Design review of the part built by this model. Coordinates are the model's own, in mm. Face numbers are marked on the shaded views. A direction names the side the tool comes from. Coordinates: 2 decimals unless noted, no trailing zeros. Write each loop counter-clockwise with the first axis right and the second up, starting at its lowest first coordinate (ties: lowest second). Pieces come first, ordered by that corner, then holes. Notation, with made-up numbers: (73.25, 4.5) - (102.25, 4.5) arc R10 ccw to (102.25, 15.5) - close; hole circle Ø1 at (65.25, 88.25). An arc over 180 degrees is marked (long way). Use a Markdown table: item, result.
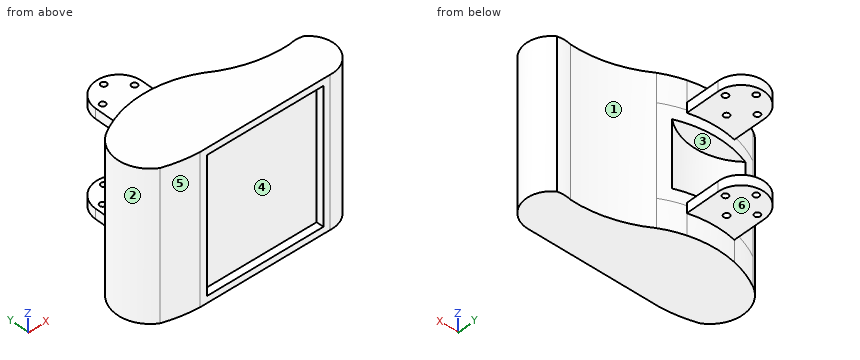
from build123d import *

# Parameters (mm, degrees)
BOSS_EXTRUDE1_DEPTH = 40
BOSS_EXTRUDE2_START = -1.2
BOSS_EXTRUDE2_DEPTH = 4.375
CUT_EXTRUDE2_START  = -29
CUT_EXTRUDE2_DEPTH  = 29
SKETCH10_R          = 1.25
CUT_EXTRUDE4_DEPTH  = 10
BOSS_EXTRUDE3_DEPTH = 12.5
SKETCH5_W           = 51.025429481
SKETCH5_H           = 59
CUT_EXTRUDE3_DEPTH  = 3.175


with BuildPart() as part:
    # Sketch1 → Boss-Extrude1 (new body)
    with BuildSketch(Plane.XY):
        with BuildLine():
            Line((-15, -2.886329782), (42.025429481, -2.886329782))
            ThreePointArc((42.025429481, -2.886329782), (53.05879951, 4.537892473), (48.73397068, 17.113670218))
            ThreePointArc((48.73397068, 17.113670218), (45.721020148, 17.497008544), (42.708069616, 17.113670218))
            ThreePointArc((42.708069616, 17.113670218), (27.113259503, 18.919115101), (12.833158081, 25.441111501))
            ThreePointArc((12.833158081, 25.441111501), (-8.642012727, 30.909979938), (-30, 25))
            ThreePointArc((-30, 25), (-37.166841919, 12.5), (-30, 0))
            ThreePointArc((-30, 0), (-22.60067635, -1.966370959), (-15, -2.886329782))
        make_face()
    extrude(amount=BOSS_EXTRUDE1_DEPTH)

    # Sketch3 → Boss-Extrude2 (add)
    with BuildSketch(Plane.XY.offset(40).offset(BOSS_EXTRUDE2_START)):
        with BuildLine():
            Line((-17.166841919, 44.092125176), (-17.166841919, 16.592125176))
            Line((-17.166841919, 16.592125176), (3.120389758, 16.592125176))
            Line((3.120389758, 16.592125176), (3.120389758, 44.092125176))
            ThreePointArc((3.120389758, 44.092125176), (-7.02322608, 54.235741015), (-17.166841919, 44.092125176))
        make_face()
    boss_extrude2 = extrude(amount=BOSS_EXTRUDE2_DEPTH)

    # Sketch4 → Cut-Extrude2 (cut)
    with BuildSketch(Plane.XY.offset(34.4).offset(CUT_EXTRUDE2_START)):
        with BuildLine():
            ThreePointArc((-23.782802313, 27.999798652), (-7.894532573, 21.994601327), (8.097551753, 27.717603087))
            ThreePointArc((8.097551753, 27.717603087), (-7.81561096, 30.910577643), (-23.782802313, 27.999798652))
        make_face()
    extrude(amount=CUT_EXTRUDE2_DEPTH, mode=Mode.SUBTRACT)

    # Sketch10 → Cut-Extrude4 (cut)
    with BuildSketch(Plane.XY.offset(43.175)):
        with Locations((-7.02322608, 51.235741015)):
            Circle(SKETCH10_R)
        with Locations((-0.02322608, 44.235741015)):
            Circle(SKETCH10_R)
        with Locations((-7.02322608, 37.235741015)):
            Circle(SKETCH10_R)
        with Locations((-14.02322608, 44.235741015)):
            Circle(SKETCH10_R)
    cut_extrude4 = extrude(amount=-CUT_EXTRUDE4_DEPTH, mode=Mode.SUBTRACT)

    # Sketch6 → Boss-Extrude3 (add)
    with BuildSketch(Plane.XY.offset(40)):
        with BuildLine():
            ThreePointArc((12.833158081, 25.441111501), (8.097551753, 27.717603087), (3.120389758, 29.401717013))
            Line((3.120389758, 29.401717013), (3.120389758, 16.592125176))
            Line((3.120389758, 16.592125176), (-17.166841919, 16.592125176))
            Line((-17.166841919, 16.592125176), (-17.166841919, 29.969927353))
            ThreePointArc((-17.166841919, 29.969927353), (-23.782802313, 27.999798652), (-30, 25))
            ThreePointArc((-30, 25), (-37.166841919, 12.5), (-30, 0))
            ThreePointArc((-30, 0), (-22.60067635, -1.966370959), (-15, -2.886329782))
            Line((-15, -2.886329782), (42.025429481, -2.886329782))
            ThreePointArc((42.025429481, -2.886329782), (53.05879951, 4.537892473), (48.73397068, 17.113670218))
            ThreePointArc((48.73397068, 17.113670218), (45.721020148, 17.497008544), (42.708069616, 17.113670218))
            ThreePointArc((42.708069616, 17.113670218), (27.113259503, 18.919115101), (12.833158081, 25.441111501))
        make_face()
        with BuildLine():
            Line((3.120389758, 16.592125176), (3.120389758, 29.401717013))
            ThreePointArc((3.120389758, 29.401717013), (-6.989349265, 30.895351044), (-17.166841919, 29.969927353))
            Line((-17.166841919, 29.969927353), (-17.166841919, 16.592125176))
            Line((-17.166841919, 16.592125176), (3.120389758, 16.592125176))
        make_face()
    boss_extrude3 = extrude(amount=BOSS_EXTRUDE3_DEPTH)

    # Mirror4: Boss-Extrude3 across plane
    add(boss_extrude3.mirror(Plane(origin=(0, 0, 20), x_dir=(1, 0, 0), z_dir=(0, 0, -1))))

    # Sketch5 → Cut-Extrude3 (cut)
    with BuildSketch(Plane.XZ.offset(2.886329782)):
        with Locations((13.512714741, 20)):
            Rectangle(SKETCH5_W, SKETCH5_H)
    extrude(amount=-CUT_EXTRUDE3_DEPTH, mode=Mode.SUBTRACT)

    # Mirror5: Boss-Extrude2, Cut-Extrude4 across plane
    add(boss_extrude2.mirror(Plane(origin=(0, 0, 20), x_dir=(1, 0, 0), z_dir=(0, 0, -1))))
    add(cut_extrude4.mirror(Plane(origin=(0, 0, 20), x_dir=(1, 0, 0), z_dir=(0, 0, -1))), mode=Mode.SUBTRACT)


solid = part.part
(1) Take a section at B-B on z = 3. Write out the cut boundary in (x, y) (1 decimal), and give its area (3 significant figures).
Determined:
| item | result |
|---|---|
| outline | (-30, 0) arc R55 ccw to (-15, -2.9) - (-12, -2.9) - (-12, 0.3) - (39, 0.3) - (39, -2.9) - (42, -2.9) arc R10.9 ccw to (48.7, 17.1) arc R12 ccw to (42.7, 17.1) arc R50.3 cw to (12.8, 25.4) arc R43.2 ccw to (-30, 25) arc R14.5 ccw to start |
| area | 2,170 mm2 |
(2) Take a section at C-C on x = 35.5. Write out the cut boundary in (y, z), and give its area (3 significant figures).
Determined:
| item | result |
|---|---|
| outline | (-2.89, -12.5) - (17.33, -12.5) - (17.33, 52.5) - (-2.89, 52.5) - (-2.89, 49.5) - (0.29, 49.5) - (0.29, -9.5) - (-2.89, -9.5) - close |
| area | 1,130 mm2 |
(3) Take a section at D-D on z = 21. Write out the cut boundary in (x, y) (1 decimal), and give its area (3 significant figures).
Determined:
| item | result |
|---|---|
| outline | (-30, 0) arc R55 ccw to (-15, -2.9) - (-12, -2.9) - (-12, 0.3) - (39, 0.3) - (39, -2.9) - (42, -2.9) arc R10.9 ccw to (48.7, 17.1) arc R12 ccw to (42.7, 17.1) arc R50.3 cw to (12.8, 25.4) arc R43.2 ccw to (8.1, 27.7) arc R24.6 cw to (-23.8, 28) arc R43.2 ccw to (-30, 25) arc R14.5 ccw to start |
| area | 1,980 mm2 |
(4) Draft analysis for pull direction Z (two halves, no side actions). For the marked faces 4, 5 and 6, state which applies: +Z half, -Z half, draft (parallel to the pull), parting line (faces both ways), or undercut.
Determined:
| item | result |
|---|---|
| face 4 | undercut |
| face 5 | draft |
| face 6 | -Z half |
(5) Take a section at A-A on y = 46.5. Write out the cut boundary in (x, z) (3 decimals).
Determined:
| item | result |
|---|---|
| outline | (-16.877, -3.175) - (2.83, -3.175) - (2.83, 1.2) - (-16.877, 1.2) - close; (-16.877, 38.8) - (2.83, 38.8) - (2.83, 43.175) - (-16.877, 43.175) - close |
(6) For L1, parallel to Z at x = -11.5, y = 0; L2, parallel to Z at x = -17, y = 32 (3 decimals); L3, parallel to X at y = 15, z = 10, list the stretches that pass through material, from the lowest coordinate up. Write a range as from..to.
Determined:
| item | result |
|---|---|
| L1 | -12.5..-9.5, 49.5..52.5 |
| L2 | -3.175..1.2, 38.8..43.175 |
| L3 | -36.95..51.09 |
(7) For pin 1 (4 mm diameter, centred on y = 11, z = 34.5, fed in from +X); pin 2 (1 mm diameter, centred on y = -2, z = 28.5, fed in from +X); pin 3 (2 mm diameter, centred on x = -0.02, y = 44.24, fed in from +Z); pin 4 (6 mm diameter, centred on x = -8.5, y = 45.5, fed in from -Z) (3 decimals), all flat-tipped, find the tip position at first contact; note any pin that passes through.
Determined:
| item | result |
|---|---|
| pin 1 | x = 53.58 |
| pin 2 | x = 48.07 |
| pin 3 | through |
| pin 4 | z = -3.175 |
(8) Machinability: for the marked faces 1, 2 and 3, which of the approach directions +Z, -Z, +X, -X, +Y, -Y give a long, thin tool a straight path to every point of the face, cutting with its end or side? Answer none if there is none.
Determined:
| item | result |
|---|---|
| face 1 | +Z, -Z, +Y |
| face 2 | +Z, -Z, -X |
| face 3 | +Y |
